```python
from build123d import *

# Parameters (mm, degrees)
SKETCH1_R                                       = 36.59505
SKETCH1_W                                       = 37.6
SKETCH1_H                                       = 19
BOSS_EXTRUDE1_DEPTH                             = 1.6
BOSS_EXTRUDE2_START                             = 8.3058
SKETCH2_R                                       = 36.59505
SKETCH2_R_2                                     = 34.1249
SKETCH2_R_3                                     = 2.2225
BOSS_EXTRUDE2_DEPTH                             = 8.3058
CSK_FOR_M2_FLAT_HEAD_MACHINE_SCREW1_D           = 2.4
CSK_FOR_M2_FLAT_HEAD_MACHINE_SCREW1_CSINK_D     = 4.4
CSK_FOR_M2_FLAT_HEAD_MACHINE_SCREW1_CSINK_ANGLE = 90
FILLET1_R                                       = 1.27
BOSS_EXTRUDE3_START                             = 1.6
SKETCH5_R                                       = 36.59505
SKETCH5_R_2                                     = 35.3949
BOSS_EXTRUDE3_DEPTH                             = 1.6
CHAMFER2_SIZE                                   = 1.27
FILLET2_R                                       = 1.27


with BuildPart() as part:
    # Sketch1 → Boss-Extrude1 (new body)
    with BuildSketch(Plane(origin=(0, 0, 0), x_dir=(1, 0, 0), z_dir=(0, 1, 0))):
        with Locations(Location((0, 0, 0), (0, 0, 270))):
            Circle(SKETCH1_R)
        with BuildLine():
            Line((-28.706144728, -16.573500386), (-24.086765224, -13.906500386))
            ThreePointArc((-24.086765224, -13.906500386), (0, 27.813000772), (24.086765224, -13.906500386))
            Line((24.086765224, -13.906500386), (28.706144728, -16.573500386))
            ThreePointArc((28.706144728, -16.573500386), (0, 33.147000772), (-28.706144728, -16.573500386))
        make_face(mode=Mode.SUBTRACT)
        Rectangle(SKETCH1_W, SKETCH1_H, mode=Mode.SUBTRACT)
    extrude(amount=BOSS_EXTRUDE1_DEPTH)

    # Sketch2 → Boss-Extrude2 (add)
    # profile 1 of 3: a face of its own
    with BuildSketch(Plane.XZ.offset(BOSS_EXTRUDE2_START)):
        with Locations(Location((0, 0, 0), (0, 0, 270))):
            Circle(SKETCH2_R)
        with Locations(Location((0, 0, 0), (0, 0, 270))):
            Circle(SKETCH2_R_2, mode=Mode.SUBTRACT)
    # profile 2 of 3: a face of its own
    with BuildSketch(Plane.XZ.offset(BOSS_EXTRUDE2_START)):
        with Locations(Location((20, 13.82014, 0), (0, 0, 90))):
            Circle(SKETCH2_R_3)
    # profile 3 of 3: a face of its own
    with BuildSketch(Plane.XZ.offset(BOSS_EXTRUDE2_START)):
        with Locations(Location((-20, 13.82014, 0), (0, 0, 90))):
            Circle(SKETCH2_R_3)
    extrude(amount=-BOSS_EXTRUDE2_DEPTH)

    # CSK for M2 Flat Head Machine Screw1 (through all)
    with Locations(Plane(origin=(0, 1.6, 0), x_dir=(1, 0, 0), z_dir=(0, 1, 0))):
        with Locations((-20, -13.82014), (20, -13.82014)):
            CounterSinkHole(CSK_FOR_M2_FLAT_HEAD_MACHINE_SCREW1_D / 2, CSK_FOR_M2_FLAT_HEAD_MACHINE_SCREW1_CSINK_D / 2, counter_sink_angle=CSK_FOR_M2_FLAT_HEAD_MACHINE_SCREW1_CSINK_ANGLE)

    # Fillet1
    fillet1_edges = [part.edges().sort_by_distance(p)[0] for p in [
        (28.706144728, 0.8, 16.573500386),
        (-28.706144728, 0.8, 16.573500386),
        (-24.086765224, 0.8, 13.906500386),
        (24.086765224, 0.8, 13.906500386),
        (18.8, 0.8, -9.5),
        (-18.8, 0.8, -9.5),
        (-18.8, 0.8, 9.5),
        (18.8, 0.8, 9.5),
    ]]
    fillet(fillet1_edges, radius=FILLET1_R)

    # Sketch5 → Boss-Extrude3 (add)
    with BuildSketch(Plane.XZ.offset(8.3058).offset(BOSS_EXTRUDE3_START)):
        with Locations(Location((0, 0, 0), (0, 0, 270))):
            Circle(SKETCH5_R)
        with Locations(Location((0, 0, 0), (0, 0, 270))):
            Circle(SKETCH5_R_2, mode=Mode.SUBTRACT)
    extrude(amount=-BOSS_EXTRUDE3_DEPTH)

    # Chamfer2
    chamfer2_edges = [part.edges().sort_by_distance(p)[0] for p in [
        (-18.8, 1.6, 0),
        (0, 1.6, 9.5),
        (18.8, 1.6, 0),
        (0, 1.6, -9.5),
        (0, 1.6, -27.813000772),
        (26.373483072, 1.6, 15.226737551),
        (0, 1.6, -33.147000772),
        (-26.373483072, 1.6, 15.226737551),
        (-18.428025612, 1.6, 9.128025612),
        (18.428025612, 1.6, 9.128025612),
        (18.428025612, 1.6, -9.128025612),
        (-18.428025612, 1.6, -9.128025612),
        (24.57833714, 1.6, 13.783189465),
        (28.572450915, 1.6, 16.04592687),
        (-28.572450915, 1.6, 16.04592687),
        (-24.57833714, 1.6, 13.783189465),
    ]]
    chamfer(chamfer2_edges, length=CHAMFER2_SIZE)

    # Fillet2
    fillet2_edges = [part.edges().sort_by_distance(p)[0] for p in [
        (0, 1.6, -36.59505),
    ]]
    fillet(fillet2_edges, radius=FILLET2_R)


solid = part.part
```
Work out the finished part from the listing and answer in its coordinate system (mm). A direction names the side the tool comes from. Give positions to 0.01 mm unless a question says otherwise; leave off trailing zeros. Loops run counter-clockwise (first coordinate to the right, second up) from the corner with the lowest first, then second, coordinate; pieces in that order, holes last. Notation, with made-up numbers: (-20, 55.25) -> (-3, 55.25) arc R15 cw to (-3, 74.25) -> close; hole circle Ø10 at (56, 64.5). An arc over 180 degrees is marked (long way). Use CSV: the item, a comma, the result in double quotes.
1. Flat-ended cylindrical pins translate along their axes: pin 1 Ø20.5 at (x, z) = (-0.5, 4) entering from -Y; pin 2 Ø5 at (y, z) = (-5.5, -6.5) entering from -X; pin 3 Ø12 at (x, z) = (22.5, 18) entering from -Y; pin 4 Ø12 at (x, z) = (11.5, -3) entering from +Y. Find the tip coordinate at first contact, or state that the pin passes through.
Found:
pin 1,"y = 0"
pin 2,"x = -36.38"
pin 3,"y = -8.31"
pin 4,"through"
2. A tool of negligible diameter and unlimited length cuts with its end or side. For faces 1 (the conical face through (18.757, 0.815, -9.485)), 2 (the cylindrical face through (-19.84, -3.92, 12.63)), 3 (the flat face through (-19, -8.306, 15)), from which of +Z, -Z, +X, -X, +Y, -Y can it reach the whole face along a straight path? Write none if from no direction.
Found:
face 1,"+Y"
face 2,"+Y, -Y"
face 3,"-Y"
3. Straight lines are drawn through the part: line 1 (Z direction, x = 0, y = 0.15); line 2 (X direction, y = 0.35, z = 0); line 3 (X direction, y = 0.15, z = 0). For each, find the intervals that lie inside material, in ascending order.
Found:
line 1,"-36.6 to -33.15, -27.81 to -9.5, 9.5 to 36.6"
line 2,"-36.59 to -33.17, -27.79 to -18.82, 18.82 to 27.79, 33.17 to 36.59"
line 3,"-36.6 to -33.15, -27.81 to -18.8, 18.8 to 27.81, 33.15 to 36.6"
4. The part is cut by section B-B (z = 0). State how many separate pieces and enclosed holes the cut face has, then the cut area to 3 significant figures.
Found:
separate pieces,"4"
enclosed holes,"0"
area,"79.2 mm^2"
5. The part is cut by section A-A (y = -6.5). Write down the section's boundary in (x, z) (1 decimal).
Found:
outline,"circle Ø73.2 at (0, 0); circle Ø4.4 at (-20, 13.8); circle Ø4.4 at (20, 13.8); hole circle Ø68.2 at (0, 0); hole circle Ø2.4 at (-20, 13.8); hole circle Ø2.4 at (20, 13.8)"
6. The part is cut by section C-C (x = 0). Write down the section's boundary in (y, z).
Found:
outline,"(-9.91, -36.6) -> (0.33, -36.6) arc R1.27 ccw to (1.6, -35.33) -> (1.6, -34.42) -> (0.33, -33.15) -> (0, -33.15) -> (0, -34.12) -> (-8.31, -34.12) -> (-8.31, -35.39) -> (-9.91, -35.39) -> close; (-9.91, 35.39) -> (-8.31, 35.39) -> (-8.31, 34.12) -> (0, 34.12) -> (0, 9.5) -> (0.33, 9.5) -> (1.6, 10.77) -> (1.6, 35.33) arc R1.27 ccw to (0.33, 36.6) -> (-9.91, 36.6) -> close; (0, -27.81) -> (0.33, -27.81) -> (1.6, -26.54) -> (1.6, -10.77) -> (0.33, -9.5) -> (0, -9.5) -> close"
7. The mould has two halves that part along Z. Classify faces 4 (the flat face through (0, 1.6, 15)), 5 (the cylindrical face through (10.25, -4.21, -32.55)): +Z half, -Z half, draft (parallel to the pull), parting line (faces both ways), or undercut.
Found:
face 4,"draft"
face 5,"undercut"
